Work out the finished part from the listing and answer in its coordinate system (mm). A direction names the side the tool comes from. Round coordinates to 2 decimals unless told otherwise and drop trailing zeros. Loops run counter-clockwise (first coordinate to the right, second up) from the corner with the lowest first, then second, coordinate; pieces in that order, holes last.
```python
from build123d import *

# Parameters (mm, degrees)
SKETCH_1_R          = 5
EXTRUDE_1_DEPTH     = 2
SKETCH_2_R          = 1.5
CUT_EXTRUDE_1_DEPTH = 5
SKETCH_3_R          = 4.1
SKETCH_3_R_2        = 2.54
CUT_EXTRUDE_2_DEPTH = 0.2


with BuildPart() as part:
    # 草圖1 → 填料-伸長1 (new body, symmetric)
    with BuildSketch(Plane.XY):
        Circle(SKETCH_1_R)
    extrude(amount=EXTRUDE_1_DEPTH, both=True)

    # 草圖2 → 除料-伸長1 (cut, through all)
    with BuildSketch(Plane.XY.offset(2)):
        Circle(SKETCH_2_R)
    extrude(amount=-CUT_EXTRUDE_1_DEPTH, mode=Mode.SUBTRACT)

    # 草圖3 → 除料-伸長2 (cut)
    with BuildSketch(Plane.XY.offset(2)):
        Circle(SKETCH_3_R)
        Circle(SKETCH_3_R_2, mode=Mode.SUBTRACT)
    cut_extrude_2 = extrude(amount=-CUT_EXTRUDE_2_DEPTH, mode=Mode.SUBTRACT)

    # 鏡射1: 除料-伸長2 across plane
    add(cut_extrude_2.mirror(Plane.XY), mode=Mode.SUBTRACT)


solid = part.part
```
1. Find section B-B (y = 0.75). Write down the section's boundary in (x, z), then the cut area to 3 significant figures.
Answer key:
outline: (-4.94, -2) - (-4.03, -2) - (-4.03, -1.8) - (-2.43, -1.8) - (-2.43, -2) - (-1.3, -2) - (-1.3, 2) - (-2.43, 2) - (-2.43, 1.8) - (-4.03, 1.8) - (-4.03, 2) - (-4.94, 2) - close; (1.3, -2) - (2.43, -2) - (2.43, -1.8) - (4.03, -1.8) - (4.03, -2) - (4.94, -2) - (4.94, 2) - (4.03, 2) - (4.03, 1.8) - (2.43, 1.8) - (2.43, 2) - (1.3, 2) - close
area: 27.9 mm2
2. Consider probe 1 along Y at (x, z) = (0, 1.6); probe 2 along Y at (x, z) = (0, 1.9); probe 3 along Z at (x, y) = (0.25, 3). Determine where each line is inside the solid, lowest interval first.
Answer key:
probe 1: y = -5 to -1.5, 1.5 to 5
probe 2: y = -5 to -4.1, -2.54 to -1.5, 1.5 to 2.54, 4.1 to 5
probe 3: z = -1.8 to 1.8
3. Find section D-D (y = 3.5). Write down the section's boundary in (x, z), then the cut area to 3 significant figures.
Answer key:
outline: (-3.57, -2) - (-2.14, -2) - (-2.14, -1.8) - (2.14, -1.8) - (2.14, -2) - (3.57, -2) - (3.57, 2) - (2.14, 2) - (2.14, 1.8) - (-2.14, 1.8) - (-2.14, 2) - (-3.57, 2) - close
area: 26.9 mm2
4. Given pin 1 (2 mm diameter, centred on x = -1.5, z = -1, fed in from +Y), flat-ended and moving along its own axis, determine where the tip first touches the part or whether it passes through.
Answer key:
pin 1: stops at y = 4.97
5. Find section A-A (x = 0). Write down the section's boundary in (y, z).
Answer key:
outline: (-5, -2) - (-4.1, -2) - (-4.1, -1.8) - (-2.54, -1.8) - (-2.54, -2) - (-1.5, -2) - (-1.5, 2) - (-2.54, 2) - (-2.54, 1.8) - (-4.1, 1.8) - (-4.1, 2) - (-5, 2) - close; (1.5, -2) - (2.54, -2) - (2.54, -1.8) - (4.1, -1.8) - (4.1, -2) - (5, -2) - (5, 2) - (4.1, 2) - (4.1, 1.8) - (2.54, 1.8) - (2.54, 2) - (1.5, 2) - close
6. Which of the six approach directions +Z, -Z, +X, -X, +Y, -Y give full straight-line access (tool end or side, diameter ignored) to faces 1 (the face through (-2, -2, -1.8)), 2 (the face through (-4, 2, 2))?
Answer key:
face 1: -Z
face 2: +Z, +X, -X, +Y, -Y
7. Find section C-C (x = 2). Write down the section's boundary in (y, z), then the cut area to 4 significant figures.
Answer key:
outline: (-4.58, -2) - (-3.58, -2) - (-3.58, -1.8) - (-1.57, -1.8) - (-1.57, -2) - (1.57, -2) - (1.57, -1.8) - (3.58, -1.8) - (3.58, -2) - (4.58, -2) - (4.58, 2) - (3.58, 2) - (3.58, 1.8) - (1.57, 1.8) - (1.57, 2) - (-1.57, 2) - (-1.57, 1.8) - (-3.58, 1.8) - (-3.58, 2) - (-4.58, 2) - close
area: 35.05 mm2
8. Determine the mould class of faces 3 (the face through (-2, -2, 1.8)), 4 (the face through (-4, 2, -2)), 5 (the face through (-1.08, -4.88, 0.03)) for opening direction Y: +Y half, -Y half, draft (parallel to the pull), parting line (faces both ways), or undercut.
Answer key:
face 3: undercut
face 4: draft
face 5: parting line
